Verification items for this drawing (mm, ordinates from the low corner). A direction names the side the tool comes from. Round coordinates to 2 decimals unless told otherwise and drop trailing zeros. Write each loop counter-clockwise with the first axis right and the second up, starting at its lowest first coordinate (ties: lowest second). Pieces come first, ordered by that corner, then holes. Notation, with made-up numbers: (56.5, 56) -> (62.5, 56) arc R11 ccw to (62.5, 66) -> close; hole circle Ø2 at (18, 30). An arc over 180 degrees is marked (long way). Return JSON: item names as keys, results as strings. Group by question number.
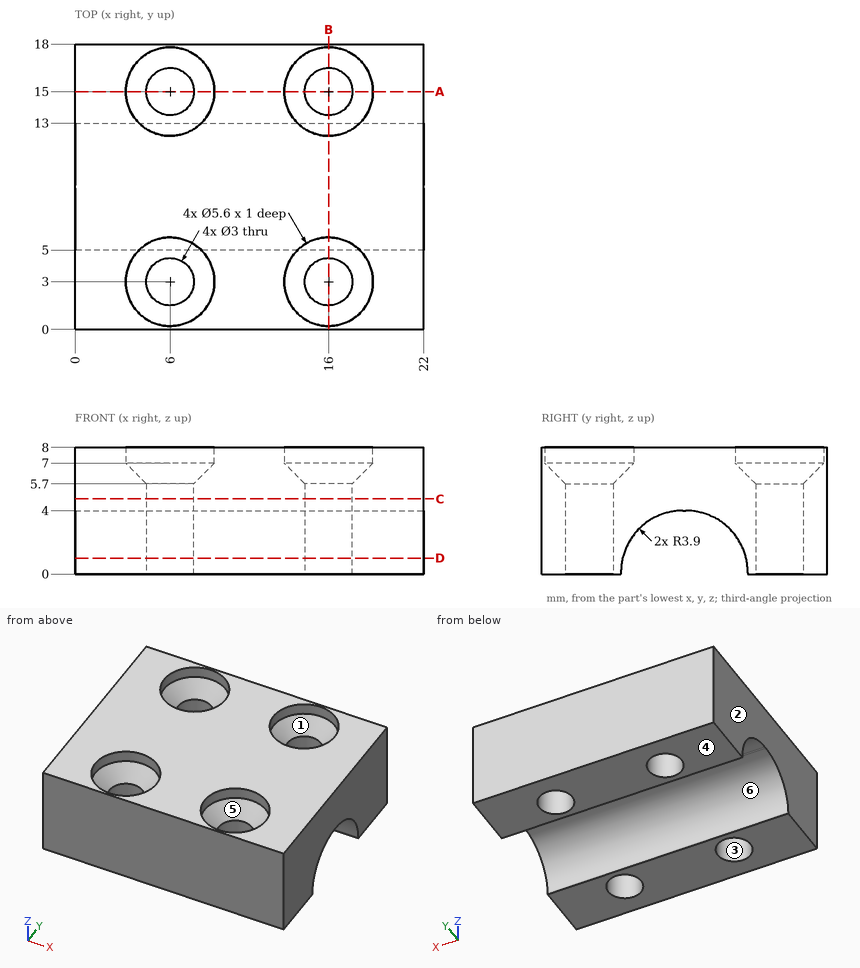
1) Sectioned sample at B-B on x = 16. Enter the section's corners in (y, z), and give its area (3 significant figures).
2) Material ranges on probe 1 along X at (y, z) = (3, 2); probe 2 along Y at (x, z) = (16, 4.2); probe 3 along Y at (x, z) = (5, 3.25), recorded low to high. Write a range as [from, to].
3) Sectioned sample at D-D on z = 1. Enter the section's corners in (x, y), and give its area (3 significant figures).
4) Sectioned sample at A-A on y = 15. Enter the section's corners in (x, z), and give its area (3 significant figures).
5) Mould release check, pull along X, two halves, no side actions. Record for the marked faces 1, 2, 3 and 4: +X half, -X half, draft (parallel to the pull), parting line (faces both ways), or undercut.
6) Sectioned sample at C-C on z = 4.75. Enter the section's corners in (x, y), and give its area (3 significant figures).
7) Tool access check on the marked faces 5 and 6. Record the directions out of +Z, -Z, +X, -X, +Y, -Y that give a thin tool (end or side, any length) a straight path to the whole face; none if there is none.
8) Go/stop test with a flat-tipped pin: P1, Ø2, axis at x = 14, y = 10, coming from the -Z side. Record where the tip stops, or that it passes through.
Evaluation:
{
 "1": {"outline": "(0, 0) -> (1.5, 0) -> (1.5, 5.7) -> (0.2, 7) -> (0.2, 8) -> (0, 8) -> close; (4.5, 0) -> (5, 0) -> (5, 0.1) arc R3.9 cw to (8.9, 4) -> (9.1, 4) arc R3.9 cw to (13, 0.1) -> (13, 0) -> (13.5, 0) -> (13.5, 5.7) -> (12.2, 7) -> (12.2, 8) -> (5.8, 8) -> (5.8, 7) -> (4.5, 5.7) -> close; (16.5, 0) -> (18, 0) -> (18, 8) -> (17.8, 8) -> (17.8, 7) -> (16.5, 5.7) -> close", "area": "61.9 mm2"},
 "2": {"probe 1": "x = [0, 4.5], [7.5, 14.5], [17.5, 22]", "probe 2": "y = [0, 1.5], [4.5, 13.5], [16.5, 18]", "probe 3": "y = [0, 1.88], [4.12, 6.6], [11.4, 13.88], [16.12, 18]"},
 "3": {"outline": "(0, 0) -> (22, 0) -> (22, 5.11) -> (0, 5.11) -> close; (0, 12.89) -> (22, 12.89) -> (22, 18) -> (0, 18) -> close; hole circle Ø3 at (6, 3); hole circle Ø3 at (6, 15); hole circle Ø3 at (16, 3); hole circle Ø3 at (16, 15)", "area": "196 mm2"},
 "4": {"outline": "(0, 0) -> (4.5, 0) -> (4.5, 5.7) -> (3.2, 7) -> (3.2, 8) -> (0, 8) -> close; (7.5, 0) -> (14.5, 0) -> (14.5, 5.7) -> (13.2, 7) -> (13.2, 8) -> (8.8, 8) -> (8.8, 7) -> (7.5, 5.7) -> close; (17.5, 0) -> (22, 0) -> (22, 8) -> (18.8, 8) -> (18.8, 7) -> (17.5, 5.7) -> close", "area": "119 mm2"},
 "5": {"face 1": "undercut", "face 2": "-X half", "face 3": "undercut", "face 4": "draft"},
 "6": {"outline": "(0, 0) -> (22, 0) -> (22, 18) -> (0, 18) -> close; hole circle Ø3 at (6, 3); hole circle Ø3 at (6, 15); hole circle Ø3 at (16, 3); hole circle Ø3 at (16, 15)", "area": "368 mm2"},
 "7": {"face 5": "+Z", "face 6": "-Z, +X, -X"},
 "8": {"P1": "stops at z = 3.51"}
}
